The listing builds one solid part. Answer for the finished solid, in the listing's coordinates (mm). Face numbers are marked on the shaded views. A direction names the side the tool comes from. Give positions to 0.01 mm unless a question says otherwise; leave off trailing zeros. Loops run counter-clockwise (first coordinate to the right, second up) from the corner with the lowest first, then second, coordinate; pieces in that order, holes last. Notation, with made-up numbers: M 76.5,-10.75 L 114.5,-10.75 A18 cw 114.5,8.25 Z; hole C 88.25,10.5 d5. An arc over 180 degrees is marked long. Use one line per item in the form item = value. Start each with the question number.
1. The part is cut by section D-D (z = 8.75). Write down the section's boundary in (x, y).
2. Straight lines are drawn through the part: line 1 (Z direction, x = 38.5, y = -2.5); line 2 (X direction, y = 3, z = 9); line 3 (X direction, y = 4.5, z = 14.5). For each, find the intervals that lie inside material, in ascending order. Write a range as from..to.
3. Each of these flat-tipped pins is pushed along its axis until it touches: pin 1 Ø4 at (y, z) = (-3, 8.5) entering from +X; pin 2 Ø2 at (x, y) = (25.5, -1.5) entering from -Z; pin 3 Ø2.5 at (x, z) = (13.5, 20.5) entering from -Y. Where does it stop, or does it pass through?
4. For the marked faces 1, 2 and 3, determine the directions among +Z, -Z, +X, -X, +Y, -Y from which every point of the face is accessible in a straight line to the end or side of a thin tool.
5. The mould has two halves that part along Z. Classify the marked faces 4, 5 and 6: released by +Z, released by -Z, zero draft, split by the parting line, or undercut.
6. The part is cut by section A-A (x = 3.5). Write down the section's boundary in (y, z), and give its area (3 significant figures).
7. The part is cut by section B-B (y = -4.25). Write down the section's boundary in (x, z), and give its area (3 significant figures).
from build123d import *

# Parameters (mm, degrees)
SKETCH_1_R           = 4
EXTRUDE_1_DEPTH      = 3
EXTRUDE_2_DEPTH      = 20
EXTRUDE_2_DEPTH_BACK = 4
SKETCH_2_R           = 4


with BuildPart() as part:
    # 草图1 → 凸台-拉伸1 (new body)
    with BuildSketch(Plane.XY):
        with BuildLine():
            Line((-6.52657961, 5.455372618), (30.448093928, 5.455372618))
            ThreePointArc((30.448093928, 5.455372618), (44.460757159, 1.735800378), (30.448093928, -1.983771861))
            Line((30.448093928, -1.983771861), (-6.52657961, -1.983771861))
            ThreePointArc((-6.52657961, -1.983771861), (-20.539242841, 1.735800378), (-6.52657961, 5.455372618))
        make_face()
        with Locations((-13.039242841, 1.735800378)):
            Circle(SKETCH_1_R, mode=Mode.SUBTRACT)
        with Locations(Location((36.960757159, 1.735800378, 0), (0, 0, 180))):
            Circle(SKETCH_1_R, mode=Mode.SUBTRACT)
    extrude_1 = extrude(amount=EXTRUDE_1_DEPTH)

    # 草图2 → 凸台-拉伸2 (add, two sides: drawn at the far end of the back side and taken through both)
    with BuildSketch(Plane.XY.offset(3).offset(-EXTRUDE_2_DEPTH_BACK)):
        with Locations((-13.039242841, 1.735800378)):
            Circle(SKETCH_2_R)
        with Locations((36.960757159, 1.735800378)):
            Circle(SKETCH_2_R)
    extrude(amount=EXTRUDE_2_DEPTH + EXTRUDE_2_DEPTH_BACK)

    # 镜向1: 凸台-拉伸1 across plane
    add(extrude_1.mirror(Plane(origin=(0, 0, 11), x_dir=(1, 0, 0), z_dir=(0, 0, -1))))


solid = part.part
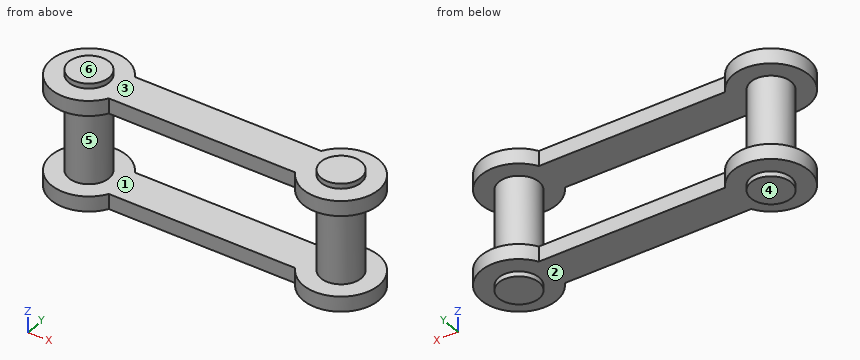
Derived:
q1.outline = C -13.04,1.74 d8; C 36.96,1.74 d8
q2.line_1 = 0..3, 19..22
q2.line_2 = -16.83..-9.24, 33.17..40.76
q2.line_3 = -15.93..-10.15, 34.07..39.85
q3.pin_1 = 39.88
q3.pin_2 = 0
q3.pin_3 = -1.98
q4.face_1 = none
q4.face_2 = -Z
q4.face_3 = +Z
q5.face_4 = released by -Z
q5.face_5 = undercut
q5.face_6 = released by +Z
q6.outline = M -1.98,0 L 5.46,0 L 5.46,3 L -1.98,3 Z; M -1.98,19 L 5.46,19 L 5.46,22 L -1.98,22 Z
q6.area = 44.6 mm2
q7.outline = M -17.56,0 L -8.52,0 L -8.52,3 L -17.56,3 Z; M -17.56,19 L -8.52,19 L -8.52,22 L -17.56,22 Z; M 32.44,0 L 41.48,0 L 41.48,3 L 32.44,3 Z; M 32.44,19 L 41.48,19 L 41.48,22 L 32.44,22 Z
q7.area = 108 mm2
